Autodesk Inventor part; units mm, degrees
ref_plane "YZ Plane" through (0, 0, 0) normal (1, 0, 0) x (0, 1, 0)
ref_plane "XZ Plane" through (0, 0, 0) normal (0, 1, 0) x (-1, 0, 0)
ref_plane "XY Plane" through (0, 0, 0) normal (0, 0, 1) x (1, 0, 0)
sketch "Sketch1" plane through (0, 0, 0) normal (0, 0, 1) x (1, 0, 0)
  line L0 (0, 0) -> (132, 0)
  line L1 (132, 0) -> (132, 30)
  line L2 (132, 30) -> (129, 30)
  line L3 (42.329, 220) -> (32.329, 218.2367)
  line L4 (32.329, 218.2367) -> (0, 0)
  line L5 (129, 30) -> (129, 22)
  line L6 (129, 22) -> (84, 5.6213)
  line L7 (84, 5.6213) -> (114.3391, 5.6213) construction
  line L8 (84, 5.6213) -> (42.329, 220)
  dimension "d0" = 132
  dimension "d1" = 220
  dimension "d3" = 3
  dimension "d4" = 8
  dimension "d6" = 20
  dimension "d7" = 81
  dimension "d8" = 10
  dimension "d9" = 10
  dimension "d20" = 30
  dimension "d22" = 45
extrude "Extrusion1" add sketch "Sketch1" along normal blind 1050
sketch "Sketch2" plane through (32.329, 218.2367, 1050) normal (-0.1736482, 0.9848078, 0) x (0.9848078, 0.1736482, 0)
  line L0 (0, 277) -> (10.1543, 277)
  line L1 (10.1543, 277) -> (10.1543, 247)
  line L2 (10.1543, 247) -> (0, 247)
  line L3 (0, 247) -> (0, 277)
  line L4 (0, 1050) -> (0, 0) construction
  line L5 (0, 803) -> (10.1543, 803)
  line L6 (10.1543, 803) -> (10.1543, 773)
  line L7 (10.1543, 773) -> (0, 773)
  line L8 (0, 773) -> (0, 803)
  line L9 (13.9657, 1050) -> (0, 1050) construction
  line L10 (10.1543, 1050) -> (10.1543, 0) construction
  point P0 (-69.7343, 1050)
  dimension "d12" = 30
  dimension "d13" = 30
  dimension "d14" = 247
  dimension "d15" = 247
extrude "Extrusion2" add sketch "Sketch2" along normal blind 220
fillet "Fillet1" radius 3 4 edges at (4.1264, 436.6577, 788) (-5.8736, 434.8944, 788) (4.1264, 436.6577, 262) (-5.8736, 434.8944, 262)
fillet "Fillet2" radius 10 4 edges at (37.329, 219.1184, 803) (37.329, 219.1184, 277) (37.329, 219.1184, 773) (37.329, 219.1184, 247)
properties part number "sostenedor1"
Can you work these out from the model? Positions are in its coordinate system, mm. A direction names the side the tool comes from. Coordinates: 2 decimals unless noted, no trailing zeros. Loops run counter-clockwise (first coordinate to the right, second up) from the corner with the lowest first, then second, coordinate; pieces in that order, holes last. Notation, with made-up numbers: M 31.5,50.5 L 69.5,50.5 A19 ccw 69.5,56.5 Z; hole C 86.25,27.25 d3. An arc over 180 degrees is marked long. Return JSON: item names as keys, results as strings. Group by question number.
Item 1: I'm going to push flat-ended pins straight in: pin 1 Ø2 at (x, z) = (106, 392.5) entering from +Y; pin 2 Ø4 at (y, z) = (26.5, 706.5) entering from -X; pin 3 Ø2 at (x, z) = (96.5, 732) entering from +Y. Where does each tip first touch, or does it pass through?
Item 2: If I drill on L1, parallel to Y at x = 108, z = 967; L2, parallel to Y at x = 86, z = 916; L3, parallel to X at y = 137.5, z = 705.5, over which ranges is the centre line in solid material (lowest first)? Write a range as from..to.
Item 3: Imagine slicing it at B-B (z = 182.5). Please give me the cut outline in (x, y), and give its area (3 significant figures).
Item 4: Imagine slicing it at D-D (y = 172). Please give me the cut outline in (x, z).
Item 5: On a 3-axis mill with a long thin cutter (end or side, diameter ignored), from which of +Z, -Z, +X, -X, +Y, -Y can I reach the whole of each face in a straight line? I mean faces 1 (the flat face through (18, 331, 247)), 2 (the flat face through (13.752, 323.592, 262.35)), 3 (the flat face through (18, 331, 803)). Say none if no direction works.
Item 6: Imagine slicing it at C-C (x = 106). Please give me the cut outline in (y, z).
Item 7: Thinking about a two-plate mould opening in Z: for faces 4 (the flat face through (50, 87, 1050)), 5 (the flat face through (18, 331, 277)), 6 (the flat face through (16.39, 110.65, 517.65)), which applies, released by +Z, released by -Z, zero draft, split by the parting line, or undercut?
Item 8: Imagine slicing it at A-A (y = 243). Please give me the cut outline in (x, z).
Verdict:
{
 "1": {"pin 1": "stops at y = 13.99", "pin 2": "stops at x = 3.63", "pin 3": "stops at y = 10.53"},
 "2": {"L1": "y = 0..14.36", "L2": "y = 0..6.35", "L3": "x = 20.37..58.37"},
 "3": {"outline": "M 0,0 L 132,0 L 132,30 L 129,30 L 129,22 L 84,5.62 L 42.33,220 L 32.33,218.24 Z", "area": "11,100 mm^2"},
 "4": {"outline": "M 25.48,0 L 51.66,0 L 51.66,1050 L 25.48,1050 Z"},
 "5": {"face 1": "-Z, +X, -X, +Y", "face 2": "+Z, -Z, -X", "face 3": "+Z, +X, -X, +Y"},
 "6": {"outline": "M 0,0 L 13.63,0 L 13.63,1050 L 0,1050 Z"},
 "7": {"face 4": "released by +Z", "face 5": "undercut", "face 6": "zero draft"},
 "8": {"outline": "M 27.96,247 L 38.27,247 L 38.27,277 L 27.96,277 Z; M 27.96,773 L 38.27,773 L 38.27,803 L 27.96,803 Z"}
}
